Can you work these out from the model? Positions are in its coordinate system, mm. A direction names the side the tool comes from. Round coordinates to 2 decimals unless told otherwise and drop trailing zeros. Order: outer loops, then holes, each group sorted by start corner. A loop starts at its lowest first (then second) coordinate and runs counter-clockwise, first axis right, second up.
Q1. If we section it at D-D (z = 3): Please give me the cut outline in (x, y), plus the area to 3 significant figures.
Q2. Will these pins go through, and if not, where does the flat tip stop? P1, Ø1.5, axis at x = 9, z = -7.5, coming from the -Y side; P2, Ø3, axis at y = 5, z = 0, coming from the -X side; P3, Ø1, axis at x = -4.5, z = -2.5, coming from the -Y side.
Q3. If I drill on line 1 (Y direction, x = 0, z = 2.85); line 2 (Z direction, x = -7.5, y = -4.5); line 3 (Y direction, x = -8, z = -9), over which ranges is the centre line in solid material (lowest first)?
Q4. If we section it at C-C (y = -14): Please give me the cut outline in (x, z).
Q5. If we section it at A-A (y = 0): Please give me the cut outline in (x, z), plus the area to 3 significant figures.
Q6. For faces 1 (the face through (7.28, -5.44, 2.55)), 2 (the face through (0, 4, 0)), which set-ups out of +Z, -Z, +X, -X, +Y, -Y let a thin tool reach every point of the face, with its end or its side?
Q7. We'd pull the mould along X, two halves only. Please class faces 3 (the face through (-13.887, -10.648, -3.888)), 4 (the face through (-14.985, 0.66, -5.916)), 5 (the face through (-3.233, 1.341, 2.028)), 6 (the face through (13, 8, -12)): pulls with the +X half, pulls with the -X half, needs draft (parallel to the pull), parting line crosses it, or undercut.
from build123d import *

# Parameters (mm, degrees)
F0_R           = 17.5
F0_R_2         = 15
F1_DEPTH       = 4
F2_DEPTH       = 12
F3_D           = 2.9
F3_CSINK_D     = 5
F3_CSINK_ANGLE = 90
F4_D           = 7


# Not quite as in the source:
# - a feature names something its author has since deleted; it is built from what else it names


with BuildPart() as f1:
    # F0 (on Top) → F1 (new body)
    with BuildSketch(Plane.XY):
        Circle(F0_R)
        Circle(F0_R_2, mode=Mode.SUBTRACT)
        Circle(F0_R_2)
    extrude(amount=F1_DEPTH)

    # F0 (on Top) → F2 (join)
    with BuildSketch(Plane.XY):
        Circle(F0_R)
        Circle(F0_R_2, mode=Mode.SUBTRACT)
    extrude(amount=-F2_DEPTH)

    # F3 (through all)
    with Locations(Plane(origin=(0, 0, 0), x_dir=(1, 0, 0), z_dir=(0, 0, -1))):
        with Locations((8.6602540378, 5), (-8.6602540378, -5)):
            CounterSinkHole(F3_D / 2, F3_CSINK_D / 2, counter_sink_angle=F3_CSINK_ANGLE)

    # F4 (through all)
    with Locations(Plane(origin=(0, 0, 0), x_dir=(1, 0, 0), z_dir=(0, 0, -1))):
        with Locations((0, 0)):
            Hole(F4_D / 2)


solid = f1.part
Solution:
1. outline: circle Ø35 at (0, 0); hole circle Ø2.9 at (-8.66, 5); hole circle Ø7 at (0, 0); hole circle Ø2.9 at (8.66, -5)
1. area: 910 mm2
2. P1: stops at y = -15.43
2. P2: stops at x = -17.15
2. P3: stops at y = -17.04
3. line 1: y = -17.5 to -3.5, 3.5 to 17.5
3. line 2: z = 0 to 4
3. line 3: y = -15.56 to -12.69, 12.69 to 15.56
4. outline: (-10.5, -12) - (-5.39, -12) - (-5.39, 0) - (5.39, 0) - (5.39, -12) - (10.5, -12) - (10.5, 4) - (-10.5, 4) - close
5. outline: (-17.5, -12) - (-15, -12) - (-15, 0) - (-3.5, 0) - (-3.5, 4) - (-17.5, 4) - close; (3.5, 0) - (15, 0) - (15, -12) - (17.5, -12) - (17.5, 4) - (3.5, 4) - close
5. area: 172 mm2
6. face 1: +Z, -Z
6. face 2: -Z
7. face 3: parting line crosses it
7. face 4: undercut
7. face 5: undercut
7. face 6: needs draft
